Autodesk Inventor part; units mm, degrees
ref_plane "YZ Plane" through (0, 0, 0) normal (1, 0, 0) x (0, 1, 0)
ref_plane "XZ Plane" through (0, 0, 0) normal (0, 1, 0) x (-1, 0, 0)
ref_plane "XY Plane" through (0, 0, 0) normal (0, 0, 1) x (1, 0, 0)
sketch "Sketch1" plane through (0, 0, 0) normal (0, 0, 1) x (1, 0, 0)
  line L0 (0, -21.016) -> (25.4, -21.016)
  line L1 (25.4, -21.016) -> (25.4, -1.966)
  line L2 (0, -1.966) -> (0, -21.016)
  line L3 (19.05, -1.966) -> (19.05, 15.687)
  line L4 (19.05, 15.687) -> (22.225, 15.687)
  line L5 (22.225, 15.687) -> (22.225, -1.966)
  line L6 (25.4, -1.966) -> (22.225, -1.966)
  line L7 (19.05, -1.966) -> (0, -1.966)
  dimension "d0" = 19.05
  dimension "d2" = 25.4
  dimension "d3" = 3.175
  dimension "d4" = 17.653
  dimension "d22" = 3.175
extrude "Extrusion1" add sketch "Sketch1" against normal blind 3.175
sketch "Sketch2" plane through (0, 0, 0) normal (0, 0, 1) x (1, 0, 0)
  line L0 (12.7, -13.0785) -> (19.05, -13.0785)
  line L1 (19.05, -13.0785) -> (19.05, -9.9035)
  line L2 (19.05, -9.9035) -> (12.7, -9.9035)
  line L3 (12.7, -9.9035) -> (12.7, -13.0785)
  line L4 (0, -1.966) -> (0, -21.016)
  line L5 (25.4, -1.966) -> (22.225, -1.966)
  line L6 (25.4, -21.016) -> (25.4, -1.966)
  dimension "d7" = 3.175
  dimension "d10" = 6.35
  dimension "d11" = 7.9375
  dimension "d12" = 6.35
extrude "Extrusion2" add sketch "Sketch2" along normal blind 6.35
sketch "Sketch3" plane through (22.225, -1.966, 0) normal (1, 0, 0) x (0, 0, -1)
  line L0 (0, 0) -> (0, 17.653)
  line L1 (0, 0) -> (3.175, 0)
  line L2 (3.175, 17.653) -> (3.175, 0)
  line L3 (0, 17.653) -> (3.175, 17.653)
  point P0 (1.5537, 16.0528)
  dimension "d38" = 1.6002
hole "Hole1" at (22.225, 14.0868, -1.5537) direction (-1, 0, 0) diameter 1.524 end through all
sketch "Sketch4" plane through (12.7, -13.0785, 0) normal (0, -1, 0) x (1, 0, 0)
  line L0 (6.35, 0) -> (0, 0)
  line L1 (6.35, 0) -> (6.35, 6.35)
  line L2 (0, 6.35) -> (6.35, 6.35)
  line L3 (0, 0) -> (0, 6.35)
  point P0 (3.175, 3.175)
hole "Hole2" at (15.875, -13.0785, 3.175) direction (0, 1, 0) diameter 3.175 end through all
sketch "Sketch5" plane through (0, 0, -3.175) normal (0, 0, -1) x (-1, 0, 0)
  line L0 (-25.4, -21.016) -> (0, -21.016)
  line L1 (0, -21.016) -> (0, -1.966)
  line L2 (0, -1.966) -> (-19.05, -1.966)
  line L3 (-19.05, -1.966) -> (-19.05, 15.687)
  line L4 (-19.05, 15.687) -> (-22.225, 15.687)
  line L5 (-22.225, 15.687) -> (-22.225, -1.966)
  line L6 (-22.225, -1.966) -> (-25.4, -1.966)
  line L7 (-25.4, -1.966) -> (-25.4, -21.016)
  point P0 (-22.225, -11.491)
  point P1 (-5.3321, 2.987)
  dimension "d37" = 3.175
hole "Hole3" at (5.3321, 2.987, -3.175) at (22.225, -11.491, -3.175) direction (0, 0, 1) diameter 3.302 end through all
sketch "Sketch6" plane through (22.225, -1.966, 0) normal (1, 0, 0) x (0, 0, -1)
  point P0 (0, 1.966)
hole "Hole4" at (22.225, -0.3658, -1.6002) direction (-1, 0, 0) diameter 1.524 end through all
thicken "Thicken1" operation add thickness 14.478 both sides no extend neighbours yes toward (0, -1, 0) faces at (21.1667, 15.687, -1.0583)
equation "\"d11\" = -0.5 * d7 + 0.5 * d0"
properties part number "slide pivot plate"
Here's how the part is built. I have some questions about the finished solid (model axes, mm). A direction names the side the tool comes from. Give positions to 0.01 mm unless a question says otherwise; leave off trailing zeros. Loops run counter-clockwise (first coordinate to the right, second up) from the corner with the lowest first, then second, coordinate; pieces in that order, holes last. Notation, with made-up numbers: M 73.25,17 L 93.25,17 A22 ccw 93.25,27 Z; hole C -19.5,-21 d1. An arc over 180 degrees is marked long. Put each result on its own line as item: value. Start each with the question number.
(1) For faces 5 (the flat face through (12.7, -11, 3)), 6 (the flat face through (10, -1.966, -2)), 7 (the flat face through (19.05, -12, 3)), which set-ups out of +Z, -Z, +X, -X, +Y, -Y let a thin tool reach every point of the face, with its end or its side?
(2) If we mould it in two halves opening along X, with no side actions, what happens to faces 1 (the flat face through (25.4, -12, -2)), 2 (the flat face through (14, -13.078, 2)), 3 (the cylindrical face through (17.425, -11.469, 3.519)), 4 (the flat face through (0, -11, -2))? For each: +X half, -X half, draft (parallel to the pull), parting line (faces both ways), or undercut.
(3) I want a section at D-D on x = 21.25. Please give me the cut outline in (y, z) (3 decimals).
(4) I want a section at A-A on y = -11.5. State how many separate pieces and enclosed holes the cut face has, then the cut area to 3 significant figures.
(5) Will these pins go through, and if not, where does the flat tip stop? pin 1 Ø1.6 at (y, z) = (-12.5, 4.5) entering from +X; pin 2 Ø1.9 at (x, z) = (15.5, 1.5) entering from -Y; pin 3 Ø4 at (x, y) = (22.225, -11.491) entering from -Z (3 decimals); pin 4 Ø3.5 at (y, z) = (0.5, -2.5) entering from -X.
(6) I want a section at C-C on z = 2.25. Please give me the cut outline in (x, y).
(7) I need wall thicknesses on line 1 along Z through (x, y) = (18.25, -16.5) (3 decimals); line 2 along Y through (x, z) = (19, 4); line 3 along X through (y, z) = (-12.25, -1). Which ranges of each line are inside material? Lowest first, please. Write a range as [from, to].
Answer block:
1. face 5: +Z, -X, +Y, -Y
1. face 6: +Z, -Z, -X, +Y
1. face 7: +Z, +X, +Y, -Y
2. face 1: +X half
2. face 2: draft
2. face 3: undercut
2. face 4: -X half
3. outline: M -21.016,-3.175 L -12.823,-3.175 L -12.823,0 L -21.016,0 Z; M -10.159,-3.175 L 1.209,-3.175 L 1.209,0 L -10.159,0 Z; hole C -0.366,-1.6 d1.524
4. separate pieces: 2
4. enclosed holes: 1
4. area: 103 mm^2
5. pin 1: x = 19.05
5. pin 2: y = -13.08
5. pin 3: z = -3.175
5. pin 4: x = 19.05
6. outline: M 12.7,-13.08 L 14.58,-13.08 L 14.58,-9.9 L 12.7,-9.9 Z; M 17.17,-13.08 L 19.05,-13.08 L 19.05,-9.9 L 17.17,-9.9 Z
7. line 1: [-3.175, 0]
7. line 2: [-13.08, -9.9]
7. line 3: [0, 20.76], [23.69, 25.4]
